from build123d import *

# Parameters (mm, degrees)
SKETCH1_W           = 42.3
SKETCH1_H           = 42.3
BOSS_EXTRUDE1_DEPTH = 48
SKETCH2_R           = 1.5
CUT_EXTRUDE1_DEPTH  = 6
SKETCH3_R           = 11
BOSS_EXTRUDE2_DEPTH = 2
SKETCH4_R           = 2.5
BOSS_EXTRUDE3_DEPTH = 22
CHAMFER1_SIZE       = 4


with BuildPart() as part:
    # Sketch1 → Boss-Extrude1 (new body)
    with BuildSketch(Plane.XY):
        Rectangle(SKETCH1_W, SKETCH1_H)
    extrude(amount=-BOSS_EXTRUDE1_DEPTH)

    # Sketch2 → Cut-Extrude1 (cut)
    with BuildSketch(Plane.XY):
        with Locations((-15.5, 15.5)):
            Circle(SKETCH2_R)
        with Locations((15.5, 15.5)):
            Circle(SKETCH2_R)
        with Locations((15.5, -15.5)):
            Circle(SKETCH2_R)
        with Locations((-15.5, -15.5)):
            Circle(SKETCH2_R)
    extrude(amount=-CUT_EXTRUDE1_DEPTH, mode=Mode.SUBTRACT)

    # Sketch3 → Boss-Extrude2 (add)
    with BuildSketch(Plane.XY):
        Circle(SKETCH3_R)
    extrude(amount=BOSS_EXTRUDE2_DEPTH)

    # Sketch4 → Boss-Extrude3 (add)
    with BuildSketch(Plane.XY.offset(2)):
        Circle(SKETCH4_R)
    extrude(amount=BOSS_EXTRUDE3_DEPTH)

    # Chamfer1
    chamfer1_edges = [part.edges().sort_by_distance(p)[0] for p in [
        (21.15, -21.15, -24),
        (-21.15, -21.15, -24),
        (-21.15, 21.15, -24),
        (21.15, 21.15, -24),
    ]]
    chamfer(chamfer1_edges, length=CHAMFER1_SIZE)


solid = part.part
Read the model definition and answer for the solid it produces. Units are mm, in the model's axes. A direction names the side the tool comes from. Coordinates: 2 decimals unless noted, no trailing zeros. Loops run counter-clockwise (first coordinate to the right, second up) from the corner with the lowest first, then second, coordinate; pieces in that order, holes last. Notation, with made-up numbers: (42.5, 4) -> (70.5, 4) arc R17 ccw to (70.5, 22) -> close; hole circle Ø11 at (-10.5, -37). An arc over 180 degrees is marked (long way). Write item = value, one per line. Start each with the question number.
1) The part is cut by section C-C, the plane z = -7.5. Determine the outline of the cut face in (x, y).
2) The part is cut by section A-A, the plane y = -15.5. Determine the outline of the cut face in (x, z), plus the area to 3 significant figures.
3) The part is cut by section D-D, the plane x = -6. Determine the outline of the cut face in (y, z).
4) Find the intervals of material crossed by L1, parallel to Y at x = 15.5, z = -4.6; L2, parallel to Z at x = -8, y = 15.5; L3, parallel to Z at x = 4.5, y = 8, in increasing order. Write a range as from..to.
5) Given P1, Ø10, axis at x = -8, y = 6, coming from the +Z side; P2, Ø8, axis at x = -9, z = 4.5, coming from the +Y side; P3, Ø0.9, axis at x = 16, y = -15.5, coming from the +Z side, each flat-ended and moving along its own axis, determine where each tip first touches the part or whether it passes through.
6) For faces 5 (the face through (0, 0, -48)), 6 (the face through (-10, -9, 0)), determine the directions among +Z, -Z, +X, -X, +Y, -Y from which every point of the face is accessible in a straight line to the end or side of a thin tool.
7) The mould has two halves that part along Y. Classify faces 1 (the face through (19.2, -19.1, -23.7)), 2 (the face through (14, 15.57, -2.96)), 3 (the face through (19.2, 19.1, -23.7)), 4 (the face through (15, -15, -6)): pulls with the +Y half, pulls with the -Y half, needs draft (parallel to the pull), parting line crosses it, or undercut.
Result:
q1.outline = (-21.15, -17.15) -> (-17.15, -21.15) -> (17.15, -21.15) -> (21.15, -17.15) -> (21.15, 17.15) -> (17.15, 21.15) -> (-17.15, 21.15) -> (-21.15, 17.15) -> close
q2.outline = (-21.15, -48) -> (21.15, -48) -> (21.15, 0) -> (17, 0) -> (17, -6) -> (14, -6) -> (14, 0) -> (-14, 0) -> (-14, -6) -> (-17, -6) -> (-17, 0) -> (-21.15, 0) -> close
q2.area = 1,990 mm²
q3.outline = (-21.15, -48) -> (21.15, -48) -> (21.15, 0) -> (9.22, 0) -> (9.22, 2) -> (-9.22, 2) -> (-9.22, 0) -> (-21.15, 0) -> close
q4.L1 = -21.15..-17, -14..14, 17..21.15
q4.L2 = -48..0
q4.L3 = -48..2
q5.P1 = 2
q5.P2 = 9.3
q5.P3 = -6
q6.face_5 = -Z, +X, -X, +Y, -Y
q6.face_6 = +Z
q7.face_1 = pulls with the -Y half
q7.face_2 = undercut
q7.face_3 = pulls with the +Y half
q7.face_4 = undercut
